Source: CAD feature listing. Evaluate the final solid. Frame: model axes, mm. Face numbers are marked on the shaded views. A direction names the side the tool comes from. Give positions to 0.01 mm unless a question says otherwise; leave off trailing zeros. Order: outer loops, then holes, each group sorted by start corner. A loop starts at its lowest first (then second) coordinate and runs counter-clockwise, first axis right, second up. Notation, with made-up numbers: (63.5, 79) - (98.5, 79) arc R28 ccw to (98.5, 109) - close; hole circle Ø1 at (-23, 49.5). An arc over 180 degrees is marked (long way). Answer as CSV lines item,"result".
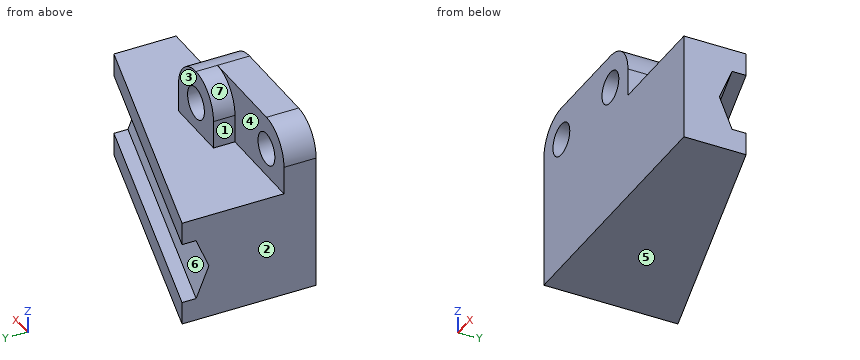
```python
from build123d import *

# Parameters (mm, degrees)
SKETCH1_W                            = 100
SKETCH1_H                            = 40
BOSS_EXTRUDE1_DEPTH                  = 50
SKETCH1_4_W                          = 35
SKETCH1_4_H                          = 23
BOSS_EXTRUDE2_DEPTH                  = 12
SKETCH1_5_W                          = 25
SKETCH1_5_H                          = 23
BOSS_EXTRUDE3_DEPTH                  = 20
FILLET1_R                            = 12.5
CUT_EXTRUDE1_DEPTH                   = 119.74342087
CUT_EXTRUDE2_DEPTH                   = 123.967511388
F_12_0_12_DIAMETER_HOLE1_D           = 12
F_12_0_12_DIAMETER_HOLE1_ON_FACE_2_D = 12


with BuildPart() as part:
    # Sketch1 → Boss-Extrude1 (new body)
    with BuildSketch(Plane(origin=(0, 0, 0), x_dir=(1, 0, 0), z_dir=(0, 1, 0))):
        with Locations((50, 20)):
            Rectangle(SKETCH1_W, SKETCH1_H)
    extrude(amount=BOSS_EXTRUDE1_DEPTH)

    # Sketch1<4> → Boss-Extrude2 (add)
    with BuildSketch(Plane(origin=(0, 0, 0), x_dir=(1, 0, 0), z_dir=(0, 1, 0))):
        with Locations((17.5, -11.5)):
            Rectangle(SKETCH1_4_W, SKETCH1_4_H)
    extrude(amount=BOSS_EXTRUDE2_DEPTH)

    # Sketch1<5> → Boss-Extrude3 (add)
    with BuildSketch(Plane(origin=(0, 0, 0), x_dir=(1, 0, 0), z_dir=(0, 1, 0))):
        with Locations((47.5, -11.5)):
            Rectangle(SKETCH1_5_W, SKETCH1_5_H)
    extrude(amount=BOSS_EXTRUDE3_DEPTH)

    # Fillet1
    fillet1_edges = [part.edges().sort_by_distance(p)[0] for p in [
        (60, 10, 23),
        (35, 16, 23),
        (0, 6, 23),
    ]]
    fillet(fillet1_edges, radius=FILLET1_R - 0.0001)  # a hair under: the kernel refuses the full size

    # Sketch2 → Cut-Extrude1 (cut, through all)
    with BuildSketch(Plane.XY):
        Polygon((0, 50), (100, 23.205080757), (100, 50), align=None)
    extrude(amount=-CUT_EXTRUDE1_DEPTH, mode=Mode.SUBTRACT)

    # Sketch4 → Cut-Extrude2 (cut, through all, along a direction that is not the sketch's normal)
    with BuildSketch(Plane.ZY):
        Polygon((-31.5, 50), (-31.5, 44.763455967), (-20, 40), (-8.5, 44.763455967), (-8.5, 50), align=None)
    extrude(amount=-CUT_EXTRUDE2_DEPTH, dir=(-0.9659258262890701, 0.2588190451025143, 0), mode=Mode.SUBTRACT)

    # Ø12.0 (12) Diameter Hole1 (through all)
    with Locations(Plane(origin=(12.5, 12, 10.5), x_dir=(0, 0, 1), z_dir=(0, 1, 0))):
        with Locations((0, 0)):
            Hole(F_12_0_12_DIAMETER_HOLE1_D / 2)

    # Ø12.0 (12) Diameter Hole1 on face 2 (through all)
    with Locations(Plane(origin=(47.5, 20, 10.5), x_dir=(0, 0, 1), z_dir=(0, 1, 0))):
        with Locations((0, 0)):
            Hole(F_12_0_12_DIAMETER_HOLE1_ON_FACE_2_D / 2)


solid = part.part
```
(1) Cut plane D-D (x = 67). Return loops of the section in (y, z), then the cut area to 3 significant figures.
Completed:
outline,"(0, -40) - (32.05, -40) - (32.05, -31.5) - (26.81, -31.5) - (22.05, -20) - (26.81, -8.5) - (32.05, -8.5) - (32.05, 0) - (0, 0) - close"
area,"1,110 mm²"
(2) Cut plane B-B (z = -1.5). Return loops of the section in (x, y).
Completed:
outline,"(0, 0) - (100, 0) - (100, 23.21) - (0, 50) - close"
(3) Ray query, line 1 (X direction, y = 7.5, z = 10.5); line 2 (Y direction, x = 38, z = 8); line 3 (Z direction, x = 21, y = 19.5). Return the intervals inside material, ascending. Write a range as from..to.
Completed:
line 1,"0..6.5, 18.5..41.5, 53.5..60"
line 2,"0..20"
line 3,"-40..0"
(4) Access query for the marked faces 1, 2 and 3. Directions: +Z, -Z, +X, -X, +Y, -Y. A direction counts if a zero-diameter tool reaches every point of the face in a straight line with its end or side. Return the directions, or none.
Completed:
face 1,"+Z, -X, +Y"
face 2,"+Z, -Z, -X, +Y, -Y"
face 3,"+Z, +X, -X, +Y"
(5) Cut plane A-A (x = 83). Return loops of the section in (y, z).
Completed:
outline,"(0, -40) - (27.76, -40) - (27.76, -31.5) - (22.52, -31.5) - (17.76, -20) - (22.52, -8.5) - (27.76, -8.5) - (27.76, 0) - (0, 0) - close"
(6) Mould query, pull axis Z, two halves, no side actions, for the marked faces 4, 5, 6 and 7. Classes: released by +Z, released by -Z, zero draft, split by the parting line, or undercut.
Completed:
face 4,"zero draft"
face 5,"released by -Z"
face 6,"undercut"
face 7,"released by +Z"
(7) Contact query for flat-ended pins moving along their axis: pin 1 (12 mm diameter, centred on x = 12.5, z = 2.5, fed in from +Y); pin 2 (3 mm diameter, centred on x = 19, y = 31, fed in from +Z); pin 3 (12 mm diameter, centred on x = 58.5, y = 18.5, fed in from +Z). Output: stop coordinate, or through.
Completed:
pin 1,"y = 48.11"
pin 2,"z = 0"
pin 3,"z = 21.96"
